Could you check a few things on this drawing? It's one solid part, dimensions in mm from its lowest x, y, z. A direction names the side the tool comes from. Give positions to 0.01 mm unless a question says otherwise; leave off trailing zeros. Loops run counter-clockwise (first coordinate to the right, second up) from the corner with the lowest first, then second, coordinate; pieces in that order, holes last. Notation, with made-up numbers: M 9.25,42 L 28.25,42 A20 ccw 28.25,80 Z; hole C 61,-28.75 d6. An arc over 180 degrees is marked long. Return JSON: item names as keys, results as strings. Group by question number.
1. For the marked faces 1, 2 and 3, which set-ups out of +Z, -Z, +X, -X, +Y, -Y let a thin tool reach every point of the face, with its end or its side?
2. If we section it at D-D (y = 70): Write out the boundary of the cut face in (x, z), plus the area to 3 significant figures.
3. Please list where these lines run through material, in increasing order: line 1 (X direction, y = 30.5, z = 70); line 2 (Z direction, x = 17.5, y = 42); line 3 (Z direction, x = 40, y = 56).
4. For pin 1 (8 mm diameter, centred on x = 22.5, y = 52, fed in from -Z); pin 2 (1 mm diameter, centred on x = 35.5, y = 22.5, fed in from -Z); pin 3 (5 mm diameter, centred on x = 26.5, y = 71, fed in from -Z), each with a flat end and sliding along its axis, tell me the tip position at first contact or that it passes through.
5. If we section it at A-A (z = 39.5): Write out the boundary of the cut face in (x, y), plus the area to 3 significant figures.
6. If we section it at C-C (x = 4.5): Write out the boundary of the cut face in (y, z), plus the area to 3 significant figures.
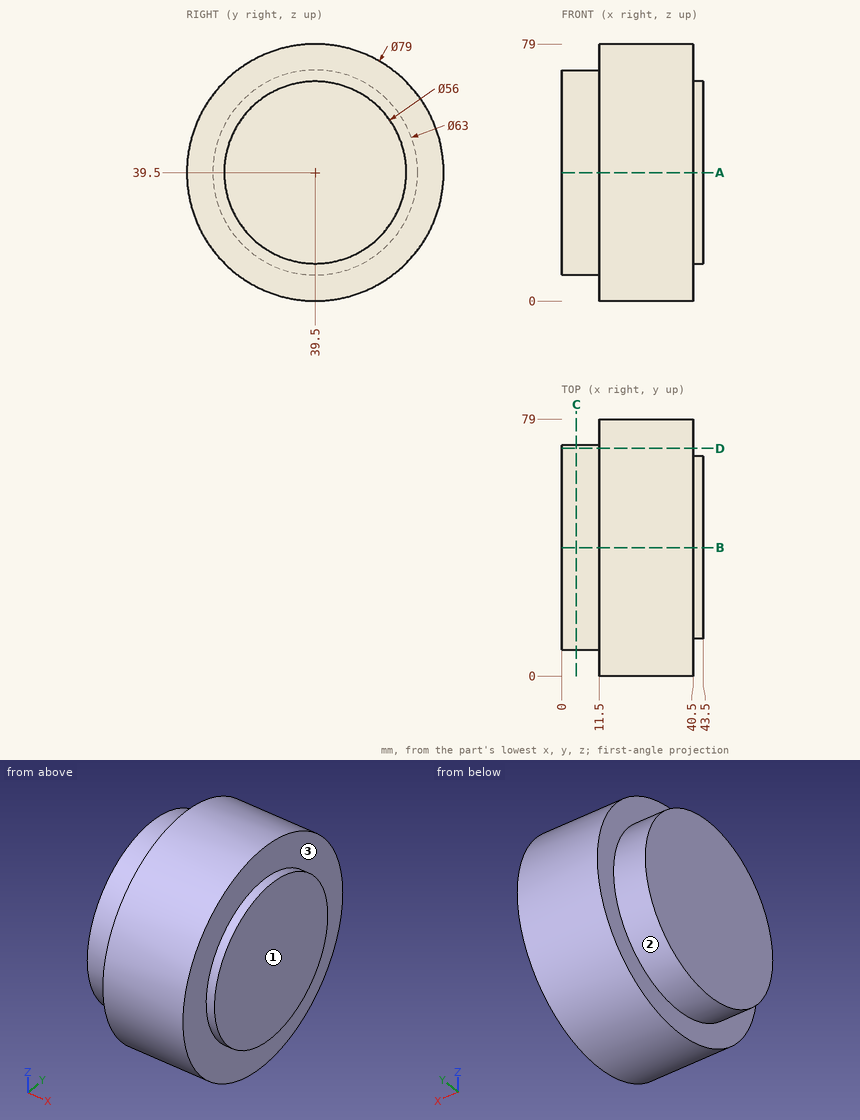
Answer:
{
 "1": {"face 1": "+Z, -Z, +X, +Y, -Y", "face 2": "-X", "face 3": "+X"},
 "2": {"outline": "M 0,31.63 L 11.5,31.63 L 11.5,14.4 L 40.5,14.4 L 40.5,64.6 L 11.5,64.6 L 11.5,47.37 L 0,47.37 Z", "area": "1,640 mm²"},
 "3": {"line 1": "x = 11.5 to 40.5", "line 2": "z = 0.08 to 78.92", "line 3": "z = 3.61 to 75.39"},
 "4": {"pin 1": "stops at z = 0.93", "pin 2": "stops at z = 3.61", "pin 3": "stops at z = 12.68"},
 "5": {"outline": "M 0,8 L 11.5,8 L 11.5,0 L 40.5,0 L 40.5,11.5 L 43.5,11.5 L 43.5,67.5 L 40.5,67.5 L 40.5,79 L 11.5,79 L 11.5,71 L 0,71 Z", "area": "3,180 mm²"},
 "6": {"outline": "C 39.5,39.5 d63", "area": "3,120 mm²"}
}
